from build123d import *

# Parameters (mm, degrees)
EXTRUDE_THIN2_DEPTH      = 5.6
BOSS_EXTRUDE1_DEPTH      = 5.6
BOSS_EXTRUDE2_DEPTH      = 5.6
BOSS_EXTRUDE2_DEPTH_BACK = 4.5
SKETCH6_R                = 5.5
FILLET1_R                = 10
SKETCH7_R                = 2.77
CUT_EXTRUDE3_DEPTH       = 4
SKETCH9_R                = 3
CUT_EXTRUDE5_DEPTH       = 3.3
SKETCH10_R               = 1.6
CUT_EXTRUDE6_DEPTH       = 26.423002314


with BuildPart() as part:
    # Sketch4 → Extrude-Thin2 (new body)
    with BuildSketch(Plane(origin=(0, 0, 0), x_dir=(1, 0, 0), z_dir=(0, 1, 0))):
        with BuildLine():
            Line((10.796856578, -1.499295844), (18.374578861, -5.874295844))
            ThreePointArc((18.374578861, -5.874295844), (19.875283017, -11.475), (14.274578861, -12.975704156))
            Line((14.274578861, -12.975704156), (6.696856578, -8.600704156))
            ThreePointArc((6.696856578, -8.600704156), (5.196152423, -3), (10.796856578, -1.499295844))
        make_face()
        with BuildLine():
            Line((9.546856578, -3.664359354), (17.124578861, -8.039359354))
            ThreePointArc((17.124578861, -8.039359354), (17.710219507, -10.225), (15.524578861, -10.810640646))
            Line((15.524578861, -10.810640646), (7.946856578, -6.435640646))
            ThreePointArc((7.946856578, -6.435640646), (7.361215932, -4.25), (9.546856578, -3.664359354))
        make_face(mode=Mode.SUBTRACT)
    extrude(amount=EXTRUDE_THIN2_DEPTH)

    # Sketch5 → Boss-Extrude1 (add)
    with BuildSketch(Plane(origin=(0, 0, 0), x_dir=(1, 0, 0), z_dir=(0, 1, 0))):
        with BuildLine():
            Line((10.796856578, -1.499295844), (2.05, 3.550704156))
            ThreePointArc((2.05, 3.550704156), (-3.550704156, 2.05), (-2.05, -3.550704156))
            Line((-2.05, -3.550704156), (6.696856578, -8.600704156))
            ThreePointArc((6.696856578, -8.600704156), (8.998238507, -9.142286296), (11.216030786, -8.323099255))
            Line((11.216030786, -8.323099255), (7.946856578, -6.435640646))
            ThreePointArc((7.946856578, -6.435640646), (7.361215932, -4.25), (9.546856578, -3.664359354))
            Line((9.546856578, -3.664359354), (12.816030786, -5.551817963))
            ThreePointArc((12.816030786, -5.551817963), (12.416571434, -3.221559989), (10.796856578, -1.499295844))
        make_face()
    extrude(amount=BOSS_EXTRUDE1_DEPTH)

    # Sketch6 → Boss-Extrude2 (add, two sides: drawn at the far end of the back side and taken through both)
    with BuildSketch(Plane(origin=(0, 0, 0), x_dir=(1, 0, 0), z_dir=(0, 1, 0)).offset(-BOSS_EXTRUDE2_DEPTH_BACK)):
        with Locations(Location((0, 0, 0), (0, 0, 270))):
            Circle(SKETCH6_R)
    extrude(amount=BOSS_EXTRUDE2_DEPTH + BOSS_EXTRUDE2_DEPTH_BACK)

    # Fillet1
    # the kernel refuses this fillet: 10 mm, written as the material it adds along each edge
    with BuildSketch(Plane(origin=(1.124901573, 5.6, 5.383734433), x_dir=(0.8660254037844402, 0, 0.4999999999999975), z_dir=(0, -1, 0))) as fillet1_piece_1:
        with BuildLine():
            CenterArc((2.77133022, 10), FILLET1_R, 245.460811273, 24.539188727)
            ThreePointArc((-1.381825119, 0.903225806), (-0.65683145, 0.503752837), (0, 0))
            Line((0, 0), (2.77133022, 0))
        make_face()
    extrude(amount=5.6)
    with BuildSketch(Plane(origin=(5.224901573, 5.6, -1.717673878), x_dir=(0.8660254037844397, 0, 0.49999999999999806), z_dir=(0, -1, 0))) as fillet1_piece_2:
        with BuildLine():
            CenterArc((2.77133022, -10), FILLET1_R, 90, 24.539188727)
            ThreePointArc((-1.381825119, -0.903225806), (-0.65683145, -0.503752837), (0, 0))
            Line((0, 0), (2.77133022, 0))
        make_face()
    extrude(amount=5.6)

    # Sketch7 → Cut-Extrude3 (cut)
    with BuildSketch(Plane.XZ.offset(4.5)):
        with Locations(Location((0, 0, 0), (0, 0, 270))):
            Circle(SKETCH7_R)
    extrude(amount=-CUT_EXTRUDE3_DEPTH, mode=Mode.SUBTRACT)

    # Sketch9 → Cut-Extrude5 (cut)
    with BuildSketch(Plane(origin=(0, 5.6, 0), x_dir=(1, 0, 0), z_dir=(0, 1, 0))):
        with Locations(Location((0, 0, 0), (0, 0, 270))):
            Circle(SKETCH9_R)
    extrude(amount=-CUT_EXTRUDE5_DEPTH, mode=Mode.SUBTRACT)

    # Sketch10 → Cut-Extrude6 (cut, through all)
    with BuildSketch(Plane(origin=(0, 2.3, 0), x_dir=(1, 0, 0), z_dir=(0, 1, 0))):
        with Locations(Location((0, 0, 0), (0, 0, 270))):
            Circle(SKETCH10_R)
    extrude(amount=-CUT_EXTRUDE6_DEPTH, mode=Mode.SUBTRACT)


solid = part.part
Verification items for the finished model (mm, model axes). A direction names the side the tool comes from. Round coordinates to 2 decimals unless told otherwise and drop trailing zeros. Order: outer loops, then holes, each group sorted by start corner. A loop starts at its lowest first (then second) coordinate and runs counter-clockwise, first axis right, second up. Notation, with made-up numbers: (25, 10.25) -> (71, 10.25) arc R11 ccw to (71, 29.25) -> close; hole circle Ø6 at (-29.75, -22). An arc over 180 degrees is marked (long way). Put each result on its own line as item: value.
1) Section check B-B (y = 3.75). Record the cut outline in (x, z) (3 decimals).
Final values:
outline: (-0.523, 5.475) arc R5.5 ccw (long way) to (4.48, -3.191) arc R10 cw to (7.625, -0.332) -> (18.375, 5.874) arc R4.1 ccw to (14.275, 12.976) -> (3.525, 6.769) arc R10 cw to start; hole circle Ø6 at (0, 0); hole (7.947, 6.436) arc R1.6 ccw to (9.547, 3.664) -> (17.125, 8.039) arc R1.6 ccw to (15.525, 10.811) -> close
2) Section check A-A (z = 0). Record the cut outline in (x, y), then the cut area to 3 significant figures.
Final values:
outline: (-5.5, -4.5) -> (-2.77, -4.5) -> (-2.77, -0.5) -> (-1.6, -0.5) -> (-1.6, 2.3) -> (-3, 2.3) -> (-3, 5.6) -> (-5.5, 5.6) -> close; (1.6, -0.5) -> (2.77, -0.5) -> (2.77, -4.5) -> (5.5, -4.5) -> (5.5, 0) -> (8.2, 0) -> (8.2, 5.6) -> (3, 5.6) -> (3, 2.3) -> (1.6, 2.3) -> close
area: 75.3 mm^2
3) Section check D-D (y = 1.5). Record the cut outline in (x, z) (3 decimals), then the cut area to 3 significant figures.
Final values:
outline: (-0.523, 5.475) arc R5.5 ccw (long way) to (4.48, -3.191) arc R10 cw to (7.625, -0.332) -> (18.375, 5.874) arc R4.1 ccw to (14.275, 12.976) -> (3.525, 6.769) arc R10 cw to start; hole circle Ø3.2 at (0, 0); hole (7.947, 6.436) arc R1.6 ccw to (9.547, 3.664) -> (17.125, 8.039) arc R1.6 ccw to (15.525, 10.811) -> close
area: 193 mm^2
4) Set-up check for faces 4 (the flat face through (-1.3, 2.3, 1.3)), 5 (the flat face through (8, 5.6, 3)), 6 (the flat face through (13.28, 2.76, 5.82)), 7 (the flat face through (-2, -0.5, 0)): record each of +Z, -Z, +X, -X, +Y, -Y from which the full face is reachable in a straight line by a thin tool's end or side.
Final values:
face 4: +Y
face 5: +Z, -Z, +X, -X, +Y
face 6: +Y, -Y
face 7: -Y
5) Material ranges on line 1 (X direction, y = -1.7, z = 0); line 2 (Y direction, x = 8.25, z = 8.75); line 3 (Z direction, x = 10.75, y = 2.25), recorded low to high.
Final values:
line 1: x = -5.5 to -2.77, 2.77 to 5.5
line 2: y = 0 to 5.6
line 3: z = 1.47 to 4.36, 8.05 to 10.94
6) Section check C-C (x = 11.25). Record the cut outline in (y, z).
Final values:
outline: (0, 1.76) -> (5.6, 1.76) -> (5.6, 4.65) -> (0, 4.65) -> close; (0, 8.34) -> (5.6, 8.34) -> (5.6, 11.23) -> (0, 11.23) -> close
7) Depth check by flat-ended pin: pin 1 (1 mm diameter, centred on x = 16, y = 4, fed in from -Z); pin 2 (5 mm diameter, centred on x = 0, z = 0, fed in from +Y); pin 3 (5 mm diameter, centred on y = 1, z = 2, fed in from +X); pin 4 (1.5 mm diameter, centred on x = 16.5, z = 3.5, fed in from +Y). Enter the tip coordinate at first touch or a pass-through.
Final values:
pin 1: stops at z = 4.21
pin 2: stops at y = 2.3
pin 3: stops at x = 15.99
pin 4: passes through
8) Mould release check, pull along Z, two halves, no side actions. Record for faces 1 (the cylindrical face through (0.9, 3.97, 2.86)), 2 (the cylindrical face through (1.542, 2.839, 5.896)), 3 (the cylindrical face through (5.921, 2.839, -1.572)): +Z half, -Z half, draft (parallel to the pull), parting line (faces both ways), or undercut.
Final values:
face 1: undercut
face 2: +Z half
face 3: -Z half
